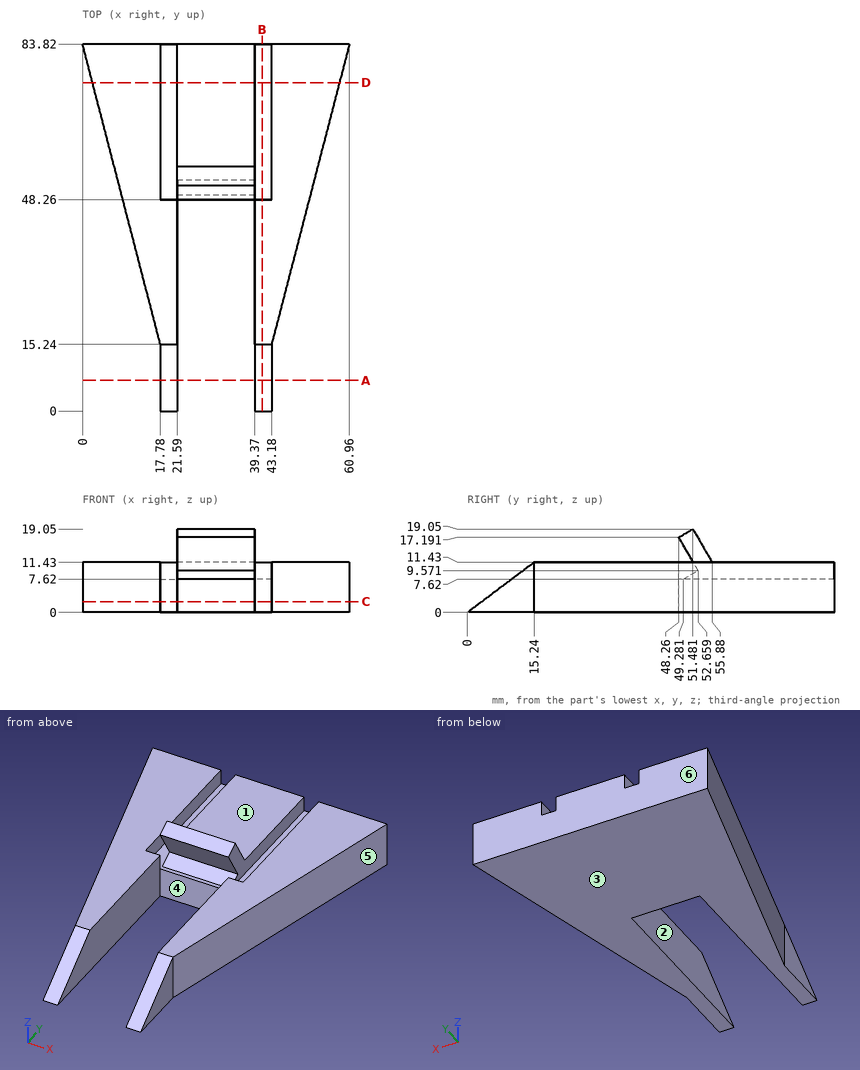
Geometry check sheet. Reference: drawing and pictorial views, mm from the part's lowest x, y, z. A direction names the side the tool comes from. Coordinates: 2 decimals unless noted, no trailing zeros. Write each loop counter-clockwise with the first axis right and the second up, starting at its lowest first coordinate (ties: lowest second). Pieces come first, ordered by that corner, then holes.
Item 1: Scan lines: probe 1 along X at (y, z) = (57, 10.5); probe 2 along Z at (x, y) = (13, 66.5); probe 3 along Z at (x, y) = (40.5, 66.5). Record each from-to range of solid material in increasing order.
Numbers:
probe 1: x = 6.95 to 17.78, 21.59 to 39.37, 43.18 to 54.01
probe 2: z = 0 to 11.43
probe 3: z = 0 to 7.62
Item 2: Cross-section at A-A on y = 7. Record the boundary of the cut face in (x, z).
Numbers:
outline: (17.78, 0) - (21.59, 0) - (21.59, 5.25) - (17.78, 5.25) - close; (39.37, 0) - (43.18, 0) - (43.18, 5.25) - (39.37, 5.25) - close
Item 3: Access from +Z, -Z, +X, -X, +Y, -Y to the whole of each face (thin tool, end or side, straight path). Record for the marked faces 1, 2 and 3.
Numbers:
face 1: +Z, +X, -X, +Y
face 2: +Z, -Z, -Y
face 3: -Z, +X, -X, +Y, -Y
Item 4: Cross-section at B-B on x = 41. Record the boundary of the cut face in (y, z).
Numbers:
outline: (0, 0) - (83.82, 0) - (83.82, 7.62) - (48.26, 7.62) - (48.26, 11.43) - (15.24, 11.43) - close
Item 5: Mould release check, pull along X, two halves, no side actions. Record for the marked faces 4, 5 and 6: released by +X, released by -X, zero draft, split by the parting line, or undercut.
Numbers:
face 4: undercut
face 5: released by +X
face 6: zero draft
Item 6: Cross-section at C-C on z = 2.5. Record the boundary of the cut face in (x, y).
Numbers:
outline: (0, 83.82) - (17.78, 15.24) - (17.78, 3.33) - (21.59, 3.33) - (21.59, 48.26) - (39.37, 48.26) - (39.37, 3.33) - (43.18, 3.33) - (43.18, 15.24) - (60.96, 83.82) - close
Item 7: Cross-section at D-D on y = 75. Record the boundary of the cut face in (x, z).
Numbers:
outline: (2.29, 0) - (58.67, 0) - (58.67, 11.43) - (43.18, 11.43) - (43.18, 7.62) - (39.37, 7.62) - (39.37, 11.43) - (21.59, 11.43) - (21.59, 7.62) - (17.78, 7.62) - (17.78, 11.43) - (2.29, 11.43) - close
Item 8: Depth check by flat-ended pin: pin 1 Ø9 at (y, z) = (6, 6.5) entering from +X; pin 2 Ø17.5 at (x, y) = (55, 60) entering from +Z; pin 3 Ø7.5 at (x, y) = (35, 58.5) entering from +Z (1 decimal). Enter the tip coordinate at first touch or a pass-through.
Numbers:
pin 1: stops at x = 43.18
pin 2: stops at z = 11.43
pin 3: stops at z = 13.4
